```python
from build123d import *

# Parameters (mm, degrees)
SKETCH1_R                         = 10
BOSS_EXTRUDE1_DEPTH               = 54.8
TAP_DRILL_FOR_M3_TAP1_D           = 2.5
TAP_DRILL_FOR_M3_TAP1_DEPTH       = 6
TAP_DRILL_FOR_M3_TAP1_CSINK_D     = 2.55
TAP_DRILL_FOR_M3_TAP1_CSINK_ANGLE = 90
TAP_DRILL_FOR_M3_TAP1_TIP         = 0.751075774
TAP_DRILL_FOR_M3_TAP2_D           = 2.5
TAP_DRILL_FOR_M3_TAP2_DEPTH       = 6
TAP_DRILL_FOR_M3_TAP2_CSINK_D     = 2.55
TAP_DRILL_FOR_M3_TAP2_CSINK_ANGLE = 90
TAP_DRILL_FOR_M3_TAP2_TIP         = 0.751075774


with BuildPart() as part:
    # Sketch1 → Boss-Extrude1 (new body)
    with BuildSketch(Plane.XY):
        with Locations(Location((0, 0, 0), (0, 0, 180))):
            Circle(SKETCH1_R)
    extrude(amount=BOSS_EXTRUDE1_DEPTH)

    # Sketch4 → Ø6.0mm Dowel Hole1 (revolve, cut)
    with BuildSketch(Plane.YZ):
        Polygon((0, 0), (0, 54.8), (3.25, 54.8), (3, 54.55), (3, 0.25), (3.25, 0), align=None)
    revolve(axis=Axis((0, 0, -6.35), (0, 0, 1)), mode=Mode.SUBTRACT)

    # Tap Drill for M3 Tap1
    with Locations(Plane(origin=(0, 0, 0), x_dir=(-1, 0, 0), z_dir=(0, 0, -1))):
        with Locations((-6.062177826, -3.5), (0, 7), (6.062177826, -3.5)):
            CounterSinkHole(TAP_DRILL_FOR_M3_TAP1_D / 2, TAP_DRILL_FOR_M3_TAP1_CSINK_D / 2, depth=TAP_DRILL_FOR_M3_TAP1_DEPTH, counter_sink_angle=TAP_DRILL_FOR_M3_TAP1_CSINK_ANGLE)
            with Locations((0, 0, -(TAP_DRILL_FOR_M3_TAP1_DEPTH + TAP_DRILL_FOR_M3_TAP1_TIP / 2))):  # 118° drill point
                Cone(0, TAP_DRILL_FOR_M3_TAP1_D / 2, TAP_DRILL_FOR_M3_TAP1_TIP, mode=Mode.SUBTRACT)

    # Tap Drill for M3 Tap2
    with Locations(Plane.XY.offset(54.8)):
        with Locations((-6.495190528, 3.75), (0, 7.5), (6.495190528, 3.75), (6.495190528, -3.75), (0, -7.5), (-6.495190528, -3.75)):
            CounterSinkHole(TAP_DRILL_FOR_M3_TAP2_D / 2, TAP_DRILL_FOR_M3_TAP2_CSINK_D / 2, depth=TAP_DRILL_FOR_M3_TAP2_DEPTH, counter_sink_angle=TAP_DRILL_FOR_M3_TAP2_CSINK_ANGLE)
            with Locations((0, 0, -(TAP_DRILL_FOR_M3_TAP2_DEPTH + TAP_DRILL_FOR_M3_TAP2_TIP / 2))):  # 118° drill point
                Cone(0, TAP_DRILL_FOR_M3_TAP2_D / 2, TAP_DRILL_FOR_M3_TAP2_TIP, mode=Mode.SUBTRACT)


solid = part.part
```
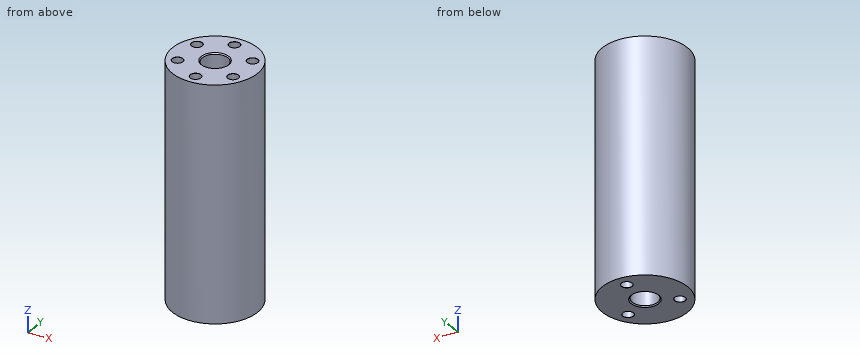
The listing builds one solid part. Answer for the finished solid, in the listing's coordinates (mm). Give positions to 0.01 mm unless a question says otherwise; leave off trailing zeros. Order: outer loops, then holes, each group sorted by start corner. A loop starts at its lowest first (then second) coordinate and runs counter-clockwise, first axis right, second up.
1) Consider line 1 along Y through (x, z) = (0, 3.45); line 2 along Y through (x, z) = (0, 51); line 3 along X through (y, z) = (-3.75, 51.95). Determine where each line is inside the solid, lowest interval first.
Reported:
line 1: y = -10 to -3, 3 to 5.75, 8.25 to 10
line 2: y = -10 to -8.75, -6.25 to -3, 3 to 6.25, 8.75 to 10
line 3: x = -9.27 to -7.75, -5.25 to 5.25, 7.75 to 9.27
2) Find section B-B on z = 22.5. Write down the section's boundary in (x, y).
Reported:
outline: circle Ø20 at (0, 0); hole circle Ø6 at (0, 0)
3) Find section C-C on z = 4. Write down the section's boundary in (x, y), then the cut area to 3 significant figures.
Reported:
outline: circle Ø20 at (0, 0); hole circle Ø2.5 at (-6.06, -3.5); hole circle Ø6 at (0, 0); hole circle Ø2.5 at (0, 7); hole circle Ø2.5 at (6.06, -3.5)
area: 271 mm2
4) Given P1, Ø3, axis at x = 6.5, y = 3.75, coming from the +Z side; P2, Ø6, axis at x = -5.5, z = 38.5, coming from the +Y side; P3, Ø2, axis at x = -6, z = 14, coming from the -Y side; P4, Ø6, axis at x = -5.5, z = 15, coming from the -Y side, each flat-ended and moving along its own axis, determine where each tip first touches the part or whether it passes through.
Reported:
P1: stops at z = 54.8
P2: stops at y = 9.68
P3: stops at y = -8.66
P4: stops at y = -9.68
5) Find section D-D on x = -3.75. Write down the section's boundary in (y, z), then the cut area to 3 significant figures.
Reported:
outline: (-9.27, 0) - (9.27, 0) - (9.27, 54.8) - (-9.27, 54.8) - close
area: 1,020 mm2
6) Find section A-A on y = 0. Write down the section's boundary in (x, z), then the cut area to 3 significant figures.
Reported:
outline: (-10, 0) - (-3.25, 0) - (-3, 0.25) - (-3, 54.55) - (-3.25, 54.8) - (-10, 54.8) - close; (3, 0.25) - (3.25, 0) - (10, 0) - (10, 54.8) - (3.25, 54.8) - (3, 54.55) - close
area: 767 mm2
